Model file for the job. Use its own axes, mm. Round coordinates to 2 decimals unless told otherwise and drop trailing zeros. Order: outer loops, then holes, each group sorted by start corner. A loop starts at its lowest first (then second) coordinate and runs counter-clockwise, first axis right, second up. Notation, with made-up numbers: (15.25, 43) - (62.25, 43) arc R27 cw to (62.25, 61) - close; hole circle Ø8 at (20.25, -12.75). An arc over 180 degrees is marked (long way). Answer as CSV lines item,"result". Start each with the question number.
1. Band-saw the part on C-C on y = 70.25. List the corners of the cut face in (x, z), then the cut area to 3 significant figures.
2. Band-saw the part on D-D on z = 26.5. State how many separate pieces and enclosed holes the cut face has, then the cut area to 3 significant figures.
3. Band-saw the part on A-A on z = 0. List the corners of the cut face in (x, y), then the cut area to 3 significant figures.
4. Pull direction X, two halves, no side cores. Call faces 1 (the face through (37.83, 67.275, 8.4)), 2 (the face through (-1, 86.401, -38)), 3 (the face through (-44.548, 82.364, 25.026)): released by +X, released by -X, zero draft, split by the parting line, or undercut.
5. Band-saw the part on B-B on y = 83.5. List the corners of the cut face in (x, z).
6. Pin check, flat tips, straight feed: pin 1 Ø4 at (x, y) = (31, 75.5) entering from +Z; pin 2 Ø4 at (y, z) = (81, 43.5) entering from +X; pin 3 Ø6.5 at (x, z) = (-45.9, 26.5) entering from -Y. Stop position of each tip, or through.
7. Wall check: line 1 along Z through (x, y) = (0, 81.25); line 2 along Z through (x, y) = (0, 78.5); line 3 along Z through (x, y) = (-45.5, 80.25). Give the ranges that are in metal, low to high. Write a range as [from, to].
```python
from build123d import *

# Parameters (mm, degrees)
SKETCH2_R          = 2
CUT_EXTRUDE1_DEPTH = 84.740671122


with BuildPart() as part:
    # Sketch1 → Revolve1 (revolve)
    with BuildSketch(Plane(origin=(0, 0, 0), x_dir=(0, 0, -1), z_dir=(1, 0, 0))):
        Polygon((37.5, 66.401492208), (57.5, 80.368434357), (57.5, 86.401492208), (37.5, 86.401492208), align=None)
    revolve(axis=Axis((0, 0, 0), (0, 1, 0)))

    # Sketch2 → Cut-Extrude1 (cut, through all)
    with BuildSketch(Plane(origin=(0, 86.401492208, 0), x_dir=(1, 0, 0), z_dir=(0, 1, 0))):
        with Locations(Location((0, -53, 0), (0, 0, 270))):
            Circle(SKETCH2_R)
        with Locations(Location((-45.899346401, -26.5, 0), (0, 0, 270))):
            Circle(SKETCH2_R)
        with Locations(Location((-45.899346401, 26.5, 0), (0, 0, 270))):
            Circle(SKETCH2_R)
        with Locations(Location((0, 53, 0), (0, 0, 270))):
            Circle(SKETCH2_R)
        with Locations(Location((45.899346401, 26.5, 0), (0, 0, 270))):
            Circle(SKETCH2_R)
        with Locations(Location((45.899346401, -26.5, 0), (0, 0, 270))):
            Circle(SKETCH2_R)
    extrude(amount=-CUT_EXTRUDE1_DEPTH, mode=Mode.SUBTRACT)


solid = part.part
```
Reply:
1,outline,"circle Ø86.02 at (0, 0); hole circle Ø75 at (0, 0)"
1,area,"1,390 mm2"
2,separate pieces,"4"
2,enclosed holes,"0"
2,area,"577 mm2"
3,outline,"(-57.5, 80.37) - (-37.5, 66.4) - (-37.5, 86.4) - (-57.5, 86.4) - close; (37.5, 66.4) - (57.5, 80.37) - (57.5, 86.4) - (37.5, 86.4) - close"
3,area,"521 mm2"
4,face 1,"split by the parting line"
4,face 2,"zero draft"
4,face 3,"undercut"
5,outline,"circle Ø115 at (0, 0); hole circle Ø4 at (-45.9, -26.5); hole circle Ø4 at (-45.9, 26.5); hole circle Ø75 at (0, 0); hole circle Ø4 at (0, -53); hole circle Ø4 at (0, 53); hole circle Ø4 at (45.9, -26.5); hole circle Ø4 at (45.9, 26.5)"
6,pin 1,"stops at z = 43.74"
6,pin 2,"stops at x = 39.8"
6,pin 3,"stops at y = 74.96"
7,line 1,"z = [-57.5, -55], [-51, -37.5], [37.5, 51], [55, 57.5]"
7,line 2,"z = [-51, -37.5], [37.5, 51]"
7,line 3,"z = [-34.88, -28.46], [-24.54, 24.54], [28.46, 34.88]"
